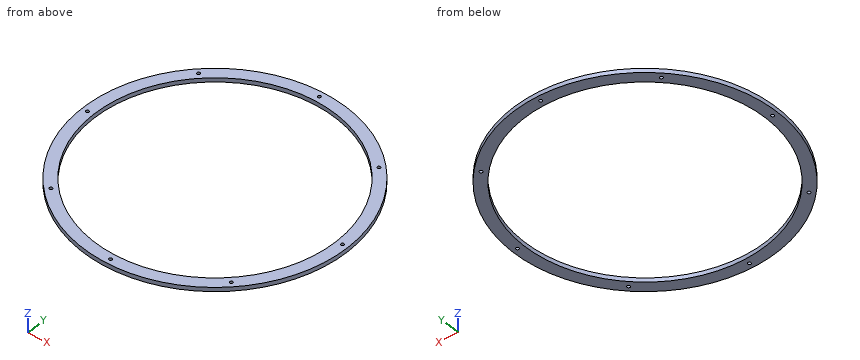
```python
from build123d import *

# Parameters (mm, degrees)
SKETCH001_R       = 95
SKETCH001_R_2     = 86.75
PAD_DEPTH         = 3
SKETCH_R          = 1.1
POCKET_DEPTH      = 3.001
POCKET_DEPTH_BACK = 0.001


with BuildPart() as part:
    # Sketch001 → Pad (new body)
    with BuildSketch(Plane(origin=(0, 0, 0), x_dir=(1, 0, 0), z_dir=(0, 0, -1))):
        Circle(SKETCH001_R)
        Circle(SKETCH001_R_2, mode=Mode.SUBTRACT)
    extrude(amount=PAD_DEPTH)

    # Sketch → Pocket (cut, two sides)
    with BuildSketch(Plane.XY) as pocket_sk:
        with Locations((64.346717, 64.346717)):
            Circle(SKETCH_R)
        with Locations((0, 91)):
            Circle(SKETCH_R)
        with Locations((91, 0)):
            Circle(SKETCH_R)
        with Locations((64.346717, -64.346717)):
            Circle(SKETCH_R)
        with Locations((0, -91)):
            Circle(SKETCH_R)
        with Locations((-91, 0)):
            Circle(SKETCH_R)
        with Locations((-64.346717, -64.346717)):
            Circle(SKETCH_R)
        with Locations((-64.346717, 64.346717)):
            Circle(SKETCH_R)
    extrude(amount=-POCKET_DEPTH, mode=Mode.SUBTRACT)
    extrude(pocket_sk.sketch, amount=POCKET_DEPTH_BACK, mode=Mode.SUBTRACT)


solid = part.part
```
Geometry: final body of the model. Coordinates: model frame, mm. Round coordinates to 2 decimals unless told otherwise and drop trailing zeros. Write each loop counter-clockwise with the first axis right and the second up, starting at its lowest first coordinate (ties: lowest second). Pieces come first, ordered by that corner, then holes. Notation, with made-up numbers: M 33.25,51 L 78.25,51 A22 ccw 78.25,81 Z; hole C 32,74.5 d9. An arc over 180 degrees is marked long. Answer in a Markdown table with one row per item. Add a question column.
(1) Ray query, L1, parallel to Y at x = 0, z = -1.3; L2, parallel to Y at x = 44.5, z = -2.55; L3, parallel to Y at x = 17, z = -0.9. Return the intervals inside material, ascending.
(2) Cut plane B-B, the plane x = -4. Return the cut outline in (y, z), then the cut area to 3 significant figures.
(3) Cut plane C-C, the plane z = -0.6. Give the number of separate pieces and of enclosed holes in the cut face, then the cut area to 3 significant figures.
(4) Cut plane A-A, the plane y = -15. Return the cut outline in (x, z), then the cut area to 3 significant figures.
(5) Contact query for flat-ended pins moving along their axis: pin 1 (1.5 mm diameter, centred on y = 33, z = -1.5, fed in from -X); pin 2 (1.5 mm diameter, centred on y = 23.5, z = -1, fed in from +X). Output: stop coordinate, or through.
Established:
| question | item | result |
|---|---|---|
| 1 | L1 | -95 to -92.1, -89.9 to -86.75, 86.75 to 89.9, 92.1 to 95 |
| 1 | L2 | -83.93 to -74.47, 74.47 to 83.93 |
| 1 | L3 | -93.47 to -85.07, 85.07 to 93.47 |
| 2 | outline | M -94.92,-3 L -86.66,-3 L -86.66,0 L -94.92,0 Z; M 86.66,-3 L 94.92,-3 L 94.92,0 L 86.66,0 Z |
| 2 | area | 49.5 mm² |
| 3 | separate pieces | 1 |
| 3 | enclosed holes | 9 |
| 3 | area | 4,680 mm² |
| 4 | outline | M -93.81,-3 L -85.44,-3 L -85.44,0 L -93.81,0 Z; M 85.44,-3 L 93.81,-3 L 93.81,0 L 85.44,0 Z |
| 4 | area | 50.2 mm² |
| 5 | pin 1 | x = -89.36 |
| 5 | pin 2 | x = 92.24 |
